Autodesk Inventor part; units mm, degrees
ref_plane "YZ Plane" through (0, 0, 0) normal (1, 0, 0) x (0, 1, 0)
ref_plane "XZ Plane" through (0, 0, 0) normal (0, 1, 0) x (-1, 0, 0)
ref_plane "XY Plane" through (0, 0, 0) normal (0, 0, 1) x (1, 0, 0)
sketch "Sketch1" plane through (0, 0, 0) normal (0, 0, 1) x (1, 0, 0)
  line L0 (7.3323, 0) -> (3.6662, -6.35)
  line L1 (3.6662, -6.35) -> (-3.6662, -6.35)
  line L2 (-3.6662, -6.35) -> (-7.3323, 0)
  line L3 (-7.3323, 0) -> (-3.6662, 6.35)
  line L4 (-3.6662, 6.35) -> (3.6662, 6.35)
  line L5 (3.6662, 6.35) -> (7.3323, 0)
  point P0 (0, 0)
  point P1 (0, 0)
  dimension "d0" = 12.7
extrude "Extrusion1" add sketch "Sketch1" along normal mid plane 76.2
sketch "Sketch2" plane through (0, 0, -38.1) normal (0, 0, -1) x (-1, 0, 0)
  circle A0 centre (0, 0) radius 15.875
  dimension "d3" = 31.75
extrude "Extrusion2" add sketch "Sketch2" along normal blind 12.7
equation "\"d0\" = printedHexSize"
equation "\"d1\" = length"
equation "\"hexSize\" = 12.7"
equation "\"slipFitOffset\" = 0"
equation "\"printedHexSize\" = hexSize - slipFitOffset"
equation "\"length\" = 76.2"
properties part number "1_2-inchHexX1_2x1_2Bushingt" material "PC/ABS Plastic"
The model under review builds one solid part; all positions refer to its coordinate system, in mm. A direction names the side the tool comes from. Round coordinates to 2 decimals unless told otherwise and drop trailing zeros. Loops run counter-clockwise (first coordinate to the right, second up) from the corner with the lowest first, then second, coordinate; pieces in that order, holes last. Notation, with made-up numbers: (68, 47) -> (91, 47) arc R21 ccw to (91, 62) -> close; hole circle Ø3 at (41.25, 73.25). An arc over 180 degrees is marked (long way). Answer in a Markdown table with one row per item.
1) Wall thickness on line 1 along Y through (x, z) = (-1, -3.5); line 2 along Z through (x, y) = (9, 9.5); line 3 along X through (y, z) = (8, -44): over which ranges is each line inside the solid? List them lowest first.
Taken from the geometry:
| item | result |
|---|---|
| line 1 | y = -6.35 to 6.35 |
| line 2 | z = -50.8 to -38.1 |
| line 3 | x = -13.71 to 13.71 |
2) Consider section C-C, the plane y = 3.5. Write out the cut boundary in (x, z).
Taken from the geometry:
| item | result |
|---|---|
| outline | (-15.48, -50.8) -> (15.48, -50.8) -> (15.48, -38.1) -> (5.31, -38.1) -> (5.31, 38.1) -> (-5.31, 38.1) -> (-5.31, -38.1) -> (-15.48, -38.1) -> close |
3) Tool access review of faces 1 (the flat face through (-5.525, 3.131, -0.533)), 2 (the flat face through (5.525, -3.131, -0.533)), 3 (the flat face through (-5.474, -3.219, -0.533)), 4 (the flat face through (0, 6.35, -1)): name each direction out of +Z, -Z, +X, -X, +Y, -Y from which nothing blocks a thin tool from reaching the whole face with its end or side.
Taken from the geometry:
| item | result |
|---|---|
| face 1 | +Z, -X, +Y |
| face 2 | +Z, +X, -Y |
| face 3 | +Z, -X, -Y |
| face 4 | +Z, +X, -X, +Y |
4) For pin 1 Ø2 at (x, z) = (-1.5, 17.5) entering from +Y; pin 2 Ø2 at (y, z) = (6, -39) entering from -X; pin 3 Ø12 at (x, z) = (-11.5, -27) entering from +Y, all flat-tipped, find the tip position at first contact; note any pin that passes through.
Taken from the geometry:
| item | result |
|---|---|
| pin 1 | stops at y = 6.35 |
| pin 2 | stops at x = -15.07 |
| pin 3 | stops at y = 3.17 |
5) Consider section A-A, the plane x = 0. Write out the cut boundary in (y, z) (3 decimals), plus the area to 3 significant figures.
Taken from the geometry:
| item | result |
|---|---|
| outline | (-15.875, -50.8) -> (15.875, -50.8) -> (15.875, -38.1) -> (6.35, -38.1) -> (6.35, 38.1) -> (-6.35, 38.1) -> (-6.35, -38.1) -> (-15.875, -38.1) -> close |
| area | 1,370 mm² |
6) Consider section B-B, the plane z = 22. Write out the cut boundary in (x, y), plus the area to 3 significant figures.
Taken from the geometry:
| item | result |
|---|---|
| outline | (-7.33, 0) -> (-3.67, -6.35) -> (3.67, -6.35) -> (7.33, 0) -> (3.67, 6.35) -> (-3.67, 6.35) -> close |
| area | 140 mm² |
7) Consider section D-D, the plane z = -43. Write out the cut boundary in (x, y) (3 decimals).
Taken from the geometry:
| item | result |
|---|---|
| outline | circle Ø31.75 at (0, 0) |
